Can you work these out from the model? Positions are in its coordinate system, mm. Face numbers are marked on the shaded views. A direction names the side the tool comes from. Give positions to 0.01 mm unless a question says otherwise; leave off trailing zeros. Write each loop counter-clockwise with the first axis right and the second up, starting at its lowest first coordinate (ties: lowest second). Pieces come first, ordered by that corner, then holes.
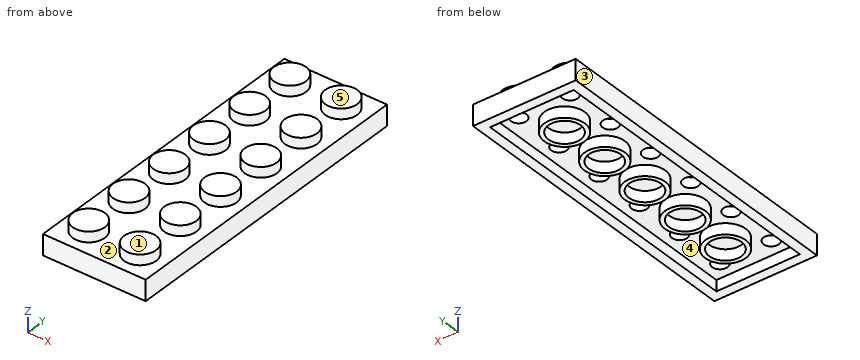
Autodesk Inventor part; units mm, degrees
ref_plane "YZ Plane" through (0, 0, 0) normal (1, 0, 0) x (0, 1, 0)
ref_plane "XZ Plane" through (0, 0, 0) normal (0, 1, 0) x (-1, 0, 0)
ref_plane "XY Plane" through (0, 0, 0) normal (0, 0, 1) x (1, 0, 0)
sketch "Sketch1" plane through (0, 0, 0) normal (0, 0, 1) x (1, 0, 0)
  line L0 (-8, 24) -> (8, 24)
  line L1 (8, 24) -> (8, -24)
  line L2 (8, -24) -> (-8, -24)
  line L3 (-8, -24) -> (-8, 24)
  point P0 (0, 0)
  dimension "d0" = 16
  dimension "d1" = 48
  dimension "d2" = 8
  dimension "d3" = 24
extrude "Extrusion1" add sketch "Sketch1" along normal blind 3.2
shell "Shell1" thickness 1.5 removed faces 1 at (-2.6667, 8, 0)
sketch "Sketch2" plane through (0, 0, 3.2) normal (0, 0, 1) x (1, 0, 0)
  circle A0 centre (4, -20) radius 2.5
  line L0 (8, 24) -> (8, -24)
  line L1 (8, -24) -> (-8, -24)
  dimension "d7" = 5
  dimension "d10" = 4
  dimension "d11" = 4
extrude "Extrusion2" add sketch "Sketch2" along normal blind 1.6
sketch "Sketch3" plane through (6.5, -22.5, 1.7) normal (0, 0, -1) x (-1, 0, 0)
  circle A0 centre (2.5, 2.5) radius 2.5
  circle A1 centre (2.5, 2.5) radius 1.2
  point P0 (6.5, 22.5)
  dimension "d18" = 2.4
extrude "Extrusion3" cut sketch "Sketch3" against normal blind 1.6 contours A1
pattern_linear "Rectangular Pattern1" count 6 spacing 8 along (0, 1, 0) count 2 spacing 8 along (-1, 0, 0) of "Extrusion2", "Extrusion3"
sketch "Sketch4" plane through (6.5, -22.5, 1.7) normal (0, 0, -1) x (-1, 0, 0)
  circle A0 centre (2.5, 10.5) radius 1.2
  circle A1 centre (2.5, 2.5) radius 1.2
  line L0 (0, 45) -> (0, 0)
  line L1 (0, 0) -> (13, 0)
  circle A2 centre (6.5, 6.5) radius 3.15
  circle A3 centre (6.5, 6.5) radius 2.5
  point P0 (6.5, 22.5)
  dimension "d21" = 6.5
  dimension "d22" = 6.5
  dimension "d23" = 10.5
  dimension "d24" = 2.5
  dimension "d25" = 5
  dimension "d26" = 6.3
extrude "Extrusion4" add sketch "Sketch4" along normal up to surface (1.7 mm away) contours A2
pattern_linear "Rectangular Pattern2" count 5 spacing 8 along (0, 1, 0) of "Extrusion4"
equation "\"d0\" = 0.8 * WIDTH"
equation "\"d1\" = 0.8 * LENGTH"
equation "\"d4\" = HEIGHT"
equation "\"d21\" = 0.5 * d23 + 0.5 * d24"
equation "\"d22\" = d21"
equation "\"WIDTH\" = 2"
equation "\"HEIGHT\" = 3.2"
properties part number "3975" material "Steel"
(1) Imagine slicing it at B-B, the plane y = 8. Write out the boundary of the cut face in (x, z).
Returned:
outline: (-8, 0) - (-6.5, 0) - (-6.5, 1.7) - (-3.15, 1.7) - (-3.15, 0) - (-2.5, 0) - (-2.5, 1.7) - (2.5, 1.7) - (2.5, 0) - (3.15, 0) - (3.15, 1.7) - (6.5, 1.7) - (6.5, 0) - (8, 0) - (8, 3.2) - (-8, 3.2) - close
(2) Will these pins go through, and if not, where does the flat tip stop? P1, Ø1.2, axis at x = 4, y = -4, coming from the -Z side; P2, Ø3, axis at x = 4, y = 4, coming from the -Z side; P3, Ø4, axis at x = 0, y = 0, coming from the +Z side; P4, Ø6, axis at x = -3.5, y = 4, coming from the -Z side.
Returned:
P1: stops at z = 3.3
P2: stops at z = 1.7
P3: stops at z = 3.2
P4: stops at z = 0
(3) Imagine slicing it at C-C, the plane y = -18. Write out the boundary of the cut face in (x, z), plus the area to 3 significant figures.
Returned:
outline: (-8, 0) - (-6.5, 0) - (-6.5, 1.7) - (-2.43, 1.7) - (-2.43, 0) - (-1.5, 0) - (-1.5, 1.7) - (1.5, 1.7) - (1.5, 0) - (2.43, 0) - (2.43, 1.7) - (6.5, 1.7) - (6.5, 0) - (8, 0) - (8, 3.2) - (5.5, 3.2) - (5.5, 4.8) - (2.5, 4.8) - (2.5, 3.2) - (-2.5, 3.2) - (-2.5, 4.8) - (-5.5, 4.8) - (-5.5, 3.2) - (-8, 3.2) - close
area: 41.9 mm2
(4) If we mould it in two halves opening along X, with no side actions, what happens to the marked faces 1, 2 and 3? For each: +X half, -X half, draft (parallel to the pull), parting line (faces both ways), or undercut.
Returned:
face 1: draft
face 2: undercut
face 3: -X half
(5) If I drill on L1, parallel to X at y = 7.5, z = 1.4; L2, parallel to X at y = -11.5, z = 1.65; L3, parallel to Y at x = 3.5, z = 0.8, over which ranges is the centre line in solid material (lowest first)?
Returned:
L1: x = -8 to -6.5, -3.11 to -2.45, 2.45 to 3.11, 6.5 to 8
L2: x = -8 to -6.5, 6.5 to 8
L3: y = -24 to -22.5, 22.5 to 24
(6) Imagine slicing it at A-A, the plane z = 0.8. Give the number of separate pieces and of enclosed holes in the cut face, plus the area to 3 significant figures.
Returned:
separate pieces: 6
enclosed holes: 6
area: 241 mm2
(7) For the marked faces 4 and 5, which set-ups out of +Z, -Z, +X, -X, +Y, -Y let a thin tool reach every point of the face, with its end or its side?
Returned:
face 4: -Z
face 5: +Z, +X, -X, +Y, -Y
